```python
from build123d import *

# Parameters (mm, degrees)
F0_R     = 35
F1_DEPTH = 5
F2_R     = 25.5
F3_DEPTH = 5
F4_R     = 1.5
F5_DEPTH = 35


with BuildPart() as f1:
    # F0 (on Front) → F1 (new body, symmetric)
    with BuildSketch(Plane.XZ):
        Circle(F0_R)
    extrude(amount=F1_DEPTH, both=True)

    # F2 (on face) → F3 (cut, symmetric)
    with BuildSketch(Plane.XZ):
        Circle(F2_R)
    extrude(amount=F3_DEPTH, both=True, mode=Mode.SUBTRACT)

    # F4 (on Top) → F5 (cut)
    with BuildSketch(Plane.XY):
        Circle(F4_R)
    extrude(amount=F5_DEPTH, mode=Mode.SUBTRACT)


solid = f1.part
```
Design review of the part built by this model. Coordinates are the model's own, in mm. Give positions to 0.01 mm unless a question says otherwise; leave off trailing zeros. Order: outer loops, then holes, each group sorted by start corner. A loop starts at its lowest first (then second) coordinate and runs counter-clockwise, first axis right, second up. Notation, with made-up numbers: M 16,-31.75 L 65,-31.75 A12 ccw 65,-22.75 Z; hole C 0.25,17 d6. An arc over 180 degrees is marked long. One line per question, with ' | ' between items. Start each with the question number.
Q1. For L1, parallel to Z at x = 0, y = -1.75; L2, parallel to Y at x = 0, z = 28; L3, parallel to X at y = 3.25, z = 1.5, list the stretches that pass through material, from the lowest coordinate up. Write a range as [from, to].
Q2. We need section A-A (z = 0). Write out the cut boundary in (x, y).
Q3. We need section B-B (x = 0). Write out the cut boundary in (y, z).
Q4. We need section C-C (y = -2.5). Write out the cut boundary in (x, z).
Q5. The part is to be moulded in two halves that separate along X. For faces 1 (the face through (-28, 0, -21)), 2 (the face through (2, 5, -26)), 3 (the face through (-1.5, 0.07, 30.16)), say which applies: +X half, -X half, draft (parallel to the pull), parting line (faces both ways), or undercut.
Q6. We need section D-D (x = 14). Write out the cut boundary in (y, z).
Q7. For pin 1 Ø1.5 at (y, z) = (2, 1) entering from -X; pin 2 Ø2 at (y, z) = (0.5, -2) entering from +X; pin 3 Ø4 at (x, y) = (-10, -3.5) entering from +Z, all flat-tipped, find the tip position at first contact; note any pin that passes through.
Returned:
1) L1: [-35, -25.5], [25.5, 35] | L2: [-5, -1.5], [1.5, 5] | L3: [-34.97, -25.46], [25.46, 34.97]
2) outline: M -35,-5 L -25.5,-5 L -25.5,5 L -35,5 Z; M 25.5,-5 L 35,-5 L 35,5 L 25.5,5 Z
3) outline: M -5,-35 L 5,-35 L 5,-25.5 L -5,-25.5 Z; M -5,25.5 L -1.5,25.5 L -1.5,35 L -5,35 Z; M 1.5,25.5 L 5,25.5 L 5,35 L 1.5,35 Z
4) outline: C 0,0 d70; hole C 0,0 d51
5) face 1: parting line | face 2: draft | face 3: undercut
6) outline: M -5,-32.08 L 5,-32.08 L 5,-21.31 L -5,-21.31 Z; M -5,21.31 L 5,21.31 L 5,32.08 L -5,32.08 Z
7) pin 1: x = -35 | pin 2: x = 34.99 | pin 3: z = 34.07
